The model under review builds one solid part; all positions refer to its coordinate system, in mm. Coordinates: 2 decimals unless noted, no trailing zeros. Write each loop counter-clockwise with the first axis right and the second up, starting at its lowest first coordinate (ties: lowest second). Pieces come first, ordered by that corner, then holes. Notation, with made-up numbers: (-28, -6.5) - (30, -6.5) arc R24 cw to (30, 15.5) - close; hole circle Ø11 at (89.5, -15.75). An arc over 180 degrees is marked (long way). Use one line per item in the form item = value. Start each with the question number.
```python
from build123d import *

# Parameters (mm, degrees)
SKETCH2_W               = 80
SKETCH2_H               = 47.65
BOSS_EXTRUDE1_DEPTH     = 3.175
SKETCH3_W               = 15
SKETCH3_H               = 3.5
BOSS_EXTRUDE2_DEPTH     = 3.175
SKETCH4_W               = 3.5
SKETCH4_H               = 15
BOSS_EXTRUDE3_DEPTH     = 3.175
MIRROR2_COPY_1_SKETCH_W = 3.5
MIRROR2_COPY_1_SKETCH_H = 15
MIRROR2_COPY_1_DEPTH    = 3.175
MIRROR2_COPY_2_SKETCH_W = 3.5
MIRROR2_COPY_2_SKETCH_H = 15
MIRROR2_COPY_2_DEPTH    = 3.175
CUT_EXTRUDE1_DEPTH      = 10
MIRROR4_COPY_1_DEPTH    = 10
CUT_EXTRUDE6_DEPTH      = 52.468303353
CUT_EXTRUDE6_DEPTH_BACK = 52.468303353
SKETCH7_R               = 1.55
CUT_EXTRUDE7_DEPTH      = 52.468303353
CUT_EXTRUDE7_DEPTH_BACK = 52.468303353


with BuildPart() as part:
    # Sketch2 → Boss-Extrude1 (new body)
    with BuildSketch(Plane(origin=(0, 0, 0), x_dir=(1, 0, 0), z_dir=(0, 1, 0))):
        Rectangle(SKETCH2_W, SKETCH2_H)
    extrude(amount=BOSS_EXTRUDE1_DEPTH)

    # Sketch3 → Boss-Extrude2 (add)
    with BuildSketch(Plane(origin=(0, 3.175, 0), x_dir=(1, 0, 0), z_dir=(0, 1, 0))):
        with Locations((0, 25.575)):
            Rectangle(SKETCH3_W, SKETCH3_H)
    boss_extrude2 = extrude(amount=-BOSS_EXTRUDE2_DEPTH)

    # Sketch4 → Boss-Extrude3 (add)
    with BuildSketch(Plane(origin=(0, 3.175, 0), x_dir=(1, 0, 0), z_dir=(0, 1, 0))):
        with Locations((-41.75, 0)):
            Rectangle(SKETCH4_W, SKETCH4_H)
    boss_extrude3 = extrude(amount=-BOSS_EXTRUDE3_DEPTH)

    # Mirror1: Boss-Extrude3 across plane
    add(boss_extrude3.mirror(Plane(origin=(0, 0, 0), x_dir=(0, 0, 1), z_dir=(1, 0, 0))))

    # Mirror2: Boss-Extrude2 across plane
    add(boss_extrude2.mirror(Plane.XY))

    # Mirror2 copy 1 sketch → Mirror2 copy 1 (add)
    with BuildSketch(Plane(origin=(0, 3.175, 0), x_dir=(-1, 0, 0), z_dir=(0, 1, 0))):
        with Locations((-41.75, 0)):
            Rectangle(MIRROR2_COPY_1_SKETCH_W, MIRROR2_COPY_1_SKETCH_H)
    extrude(amount=-MIRROR2_COPY_1_DEPTH)

    # Mirror2 copy 2 sketch → Mirror2 copy 2 (add)
    with BuildSketch(Plane(origin=(0, 3.175, 0), x_dir=(1, 0, 0), z_dir=(0, 1, 0))):
        with Locations((-41.75, 0)):
            Rectangle(MIRROR2_COPY_2_SKETCH_W, MIRROR2_COPY_2_SKETCH_H)
    extrude(amount=-MIRROR2_COPY_2_DEPTH)

    # Sketch5 → Cut-Extrude1 (cut)
    with BuildSketch(Plane(origin=(0, 3.175, 0), x_dir=(1, 0, 0), z_dir=(0, 1, 0))):
        Polygon((-40, 13.55), (-36, 13.55), (-36, 14.55), (-32.5, 14.55), (-32.5, 10.45), (-36, 10.45), (-36, 11.45), (-40, 11.45), align=None)
    cut_extrude1 = extrude(amount=-CUT_EXTRUDE1_DEPTH, mode=Mode.SUBTRACT)

    # Mirror3: Cut-Extrude1 across plane
    add(cut_extrude1.mirror(Plane.XY), mode=Mode.SUBTRACT)

    # Mirror4: Cut-Extrude1 across plane
    add(cut_extrude1.mirror(Plane(origin=(0, 0, 0), x_dir=(0, 0, 1), z_dir=(1, 0, 0))), mode=Mode.SUBTRACT)

    # Mirror4 copy 1 sketch → Mirror4 copy 1 (cut)
    with BuildSketch(Plane(origin=(0, 3.175, 0), x_dir=(-1, 0, 0), z_dir=(0, 1, 0))):
        Polygon((-40, 13.55), (-36, 13.55), (-36, 14.55), (-32.5, 14.55), (-32.5, 10.45), (-36, 10.45), (-36, 11.45), (-40, 11.45), align=None)
    extrude(amount=-MIRROR4_COPY_1_DEPTH, mode=Mode.SUBTRACT)

    # Sketch7 → Cut-Extrude6 (cut, two sides: drawn at the far end of the back side and taken through both)
    with BuildSketch(Plane(origin=(0, 0, 0), x_dir=(1, 0, 0), z_dir=(0, 1, 0)).offset(-CUT_EXTRUDE6_DEPTH_BACK)):
        with Locations(Location((0, 0, 0), (0, 0, 270))):
            Circle(SKETCH7_R)
    extrude(amount=CUT_EXTRUDE6_DEPTH + CUT_EXTRUDE6_DEPTH_BACK, mode=Mode.SUBTRACT)

    # Sketch8 → Cut-Extrude7 (cut, two sides: drawn at the far end of the back side and taken through both)
    with BuildSketch(Plane(origin=(0, 3.175, 0), x_dir=(1, 0, 0), z_dir=(0, 1, 0)).offset(-CUT_EXTRUDE7_DEPTH_BACK)):
        with BuildLine():
            Line((-22.5, 17.825), (-10, 17.825))
            ThreePointArc((-10, 17.825), (-7.171572875, 16.653427125), (-6, 13.825))
            Line((-6, 13.825), (-6, -13.825))
            ThreePointArc((-6, -13.825), (-7.171572875, -16.653427125), (-10, -17.825))
            Line((-10, -17.825), (-22.5, -17.825))
            ThreePointArc((-22.5, -17.825), (-25.328427125, -16.653427125), (-26.5, -13.825))
            Line((-26.5, -13.825), (-26.5, 13.825))
            ThreePointArc((-26.5, 13.825), (-25.328427125, 16.653427125), (-22.5, 17.825))
        make_face()
        with BuildLine():
            Line((22.5, -17.825), (10, -17.825))
            ThreePointArc((10, -17.825), (7.171572875, -16.653427125), (6, -13.825))
            Line((6, -13.825), (6, 13.825))
            ThreePointArc((6, 13.825), (7.171572875, 16.653427125), (10, 17.825))
            Line((10, 17.825), (22.5, 17.825))
            ThreePointArc((22.5, 17.825), (25.328427125, 16.653427125), (26.5, 13.825))
            Line((26.5, 13.825), (26.5, -13.825))
            ThreePointArc((26.5, -13.825), (25.328427125, -16.653427125), (22.5, -17.825))
        make_face()
    extrude(amount=CUT_EXTRUDE7_DEPTH + CUT_EXTRUDE7_DEPTH_BACK, mode=Mode.SUBTRACT)


solid = part.part
```
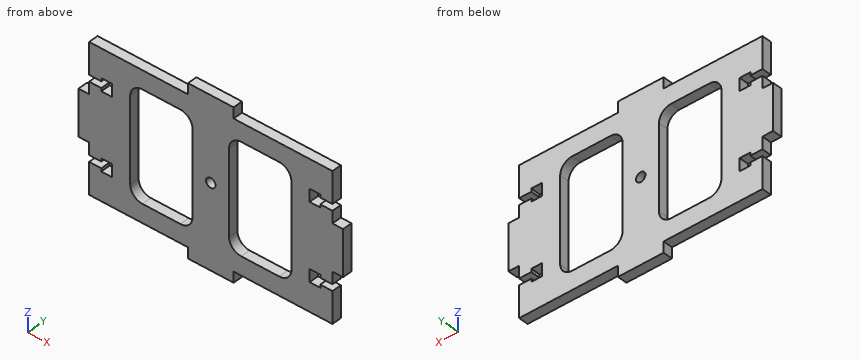
1. Take a section at C-C (x = 0). State the section outline as (y, z) points (3 decimals).
2. Take a section at D-D (y = 2). Count the separate pieces of the cut face and the enclosed holes in it, plus the area to 3 significant figures.
3. Take a section at B-B (z = 0). State the section outline as (x, y) points (3 decimals).
4. Take a section at A-A (x = -18.5). State the section outline as (y, z) points (3 decimals).
5. For P1, Ø1.6, axis at x = -13.5, y = 1, coming from the -Z side (3 decimals); P2, Ø1.6, axis at y = 1.5, z = 11.5, coming from the -X side; P3, Ø1.6, axis at x = -26, y = 2, coming from the +Z side (3 decimals), all flat-tipped, find the tip position at first contact; note any pin that passes through.
6. For L1, parallel to X at y = 1.3, z = 0; L2, parallel to Z at x = 38, y = 2.9 (3 decimals); L3, parallel to X at y = 1.4, z = -9.5, list the stretches that pass through material, from the lowest coordinate up.
Returned:
q1.outline = (0, -27.325) - (3.175, -27.325) - (3.175, -1.55) - (0, -1.55) - close; (0, 1.55) - (3.175, 1.55) - (3.175, 27.325) - (0, 27.325) - close
q2.separate_pieces = 1
q2.enclosed_holes = 3
q2.area = 2,490 mm²
q3.outline = (-43.5, 0) - (-26.5, 0) - (-26.5, 3.175) - (-43.5, 3.175) - close; (-6, 0) - (-1.55, 0) - (-1.55, 3.175) - (-6, 3.175) - close; (1.55, 0) - (6, 0) - (6, 3.175) - (1.55, 3.175) - close; (26.5, 0) - (43.5, 0) - (43.5, 3.175) - (26.5, 3.175) - close
q4.outline = (0, -23.825) - (3.175, -23.825) - (3.175, -17.825) - (0, -17.825) - close; (0, 17.825) - (3.175, 17.825) - (3.175, 23.825) - (0, 23.825) - close
q5.P1 = -23.825
q5.P2 = -40
q5.P3 = 23.825
q6.L1 = -43.5 to -26.5, -6 to -1.55, 1.55 to 6, 26.5 to 43.5
q6.L2 = -23.825 to -13.55, -11.45 to 11.45, 13.55 to 23.825
q6.L3 = -40 to -26.5, -6 to 6, 26.5 to 40
